Autodesk Inventor part; units mm, degrees
ref_plane "Work Plane1" through (0, 0, -9.525) normal (0, 0, -1) x (-1, 0, 0)
ref_plane "YZ Plane" through (0, 0, 0) normal (1, 0, 0) x (0, 1, 0)
ref_plane "XZ Plane" through (0, 0, 0) normal (0, 1, 0) x (-1, 0, 0)
sketch "Sketch1" plane through (0, 0, 0) normal (0, 0, 1) x (1, 0, 0)
  line L0 (-7.62, 3.048) -> (7.62, 3.048)
  line L1 (7.62, 3.048) -> (7.62, -3.048)
  line L2 (7.62, -3.048) -> (-7.62, -3.048)
  line L3 (-7.62, -3.048) -> (-7.62, 3.048)
  point P0 (0, 0)
  point P1 (0, -3.048)
  point P2 (-7.62, 0)
  dimension "d0" = 15.24
  dimension "d1" = 6.096
extrude "Extrusion1" add sketch "Sketch1" along normal blind 15.24
sketch "Sketch2" plane through (-7.62, 3.048, 0) normal (0, 1, 0) x (1, 0, 0)
  line L0 (0, -15.24) -> (15.24, -15.24)
  line L1 (2.54, -13.208) -> (12.7, -13.208)
  line L2 (12.7, -13.208) -> (12.7, -15.24)
  line L3 (12.7, -15.24) -> (2.54, -15.24)
  line L4 (2.54, -15.24) -> (2.54, -13.208)
  point P0 (7.62, -15.24)
  dimension "d4" = 10.16
  dimension "d5" = 2.032
extrude "Extrusion2" add sketch "Sketch2" along normal blind 1.27
sketch "Sketch3" plane through (-7.62, -3.048, 0) normal (0, -1, 0) x (1, 0, 0)
  line L0 (0, 15.24) -> (2.54, 15.24)
  line L1 (2.54, 15.24) -> (2.54, 13.208)
  line L2 (2.54, 13.208) -> (0, 13.208)
  line L3 (0, 13.208) -> (0, 15.24)
  line L4 (15.24, 15.24) -> (12.7, 15.24)
  line L5 (12.7, 15.24) -> (12.7, 13.208)
  line L6 (12.7, 13.208) -> (15.24, 13.208)
  line L7 (15.24, 13.208) -> (15.24, 15.24)
  dimension "d8" = 2.54
  dimension "d9" = 2.54
  dimension "d10" = 2.032
  dimension "d11" = 2.032
extrude "Extrusion3" add sketch "Sketch3" along normal blind 0.508
sketch "Sketch4" plane through (0, 0, 0) normal (0, 0, -1) x (-1, 0, 0)
  line L0 (7.62, 3.048) -> (-7.62, 3.048)
  line L1 (-7.62, 3.048) -> (-7.62, -3.048)
  line L2 (-7.62, -3.048) -> (7.62, -3.048)
  line L3 (7.62, -3.048) -> (7.62, 3.048)
  point P0 (-6.35, 1.27)
  point P1 (-3.81, 1.27)
  point P2 (3.81, 1.27)
  point P3 (6.35, 1.27)
  point P4 (-6.35, -1.27)
  point P5 (-3.81, -1.27)
  point P6 (3.81, -1.27)
  point P7 (6.35, -1.27)
  point P8 (0, 3.048)
  point P9 (-1.27, 1.27)
  point P10 (-1.27, -1.27)
  point P11 (1.27, 1.27)
  point P12 (1.27, -1.27)
  dimension "d14" = 1.27
  dimension "d15" = 1.778
  dimension "d16" = 1.27
  dimension "d17" = 1.778
  dimension "d18" = 2.54
  dimension "d19" = 2.54
  dimension "d20" = 2.54
  dimension "d21" = 2.54
ref_plane "Work Plane1" through (0, 0, -9.525) normal (0, 0, -1) x (-1, 0, 0)
sketch "Sketch5" plane through (0, 0, -9.525) normal (0, 0, -1) x (-1, 0, 0)
  point P0 (0, 0)
properties part number "12 Pin DR"
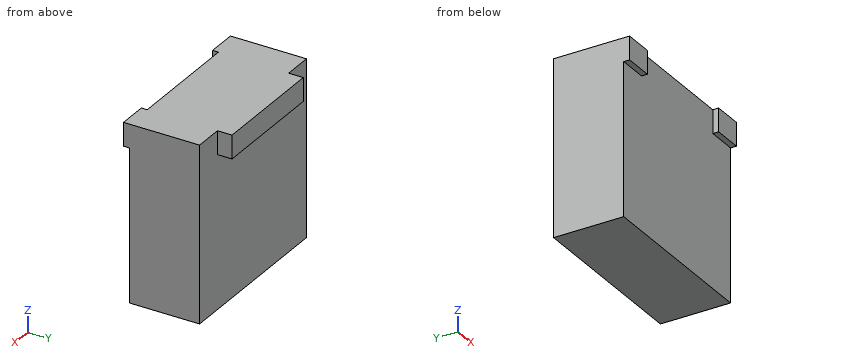
Work out the finished part from the listing and answer in its coordinate system (mm). Coordinates: 2 decimals unless noted, no trailing zeros. Loops run counter-clockwise (first coordinate to the right, second up) from the corner with the lowest first, then second, coordinate; pieces in that order, holes last. Notation, with made-up numbers: (-29.75, 53) - (-12.75, 53) arc R15 ccw to (-12.75, 72) - close; hole circle Ø6 at (-37, 75.5). An arc over 180 degrees is marked (long way). Use a Markdown table: item, result.
Item 1: Find section D-D, the plane z = 7. Determine the outline of the cut face in (x, y), and give its area (3 significant figures).
Evaluation:
| item | result |
|---|---|
| outline | (-7.62, -3.05) - (7.62, -3.05) - (7.62, 3.05) - (-7.62, 3.05) - close |
| area | 92.9 mm2 |
Item 2: Given pin 1 Ø3 at (x, y) = (-6, 2) entering from -Z; pin 2 Ø2 at (x, z) = (-1, 5.5) entering from -Y; pin 3 Ø0.6 at (y, z) = (3.5, 14) entering from -X; pin 4 Ø3 at (x, z) = (-5, 10) entering from +Y, each flat-ended and moving along its own axis, determine where each tip first touches the part or whether it passes through.
Evaluation:
| item | result |
|---|---|
| pin 1 | stops at z = 0 |
| pin 2 | stops at y = -3.05 |
| pin 3 | stops at x = -5.08 |
| pin 4 | stops at y = 3.05 |
Item 3: Find section C-C, the plane y = 3.75. Determine the outline of the cut face in (x, z).
Evaluation:
| item | result |
|---|---|
| outline | (-5.08, 13.21) - (5.08, 13.21) - (5.08, 15.24) - (-5.08, 15.24) - close |
Item 4: Find section B-B, the plane z = 14. Determine the outline of the cut face in (x, y).
Evaluation:
| item | result |
|---|---|
| outline | (-7.62, -3.56) - (-5.08, -3.56) - (-5.08, -3.05) - (5.08, -3.05) - (5.08, -3.56) - (7.62, -3.56) - (7.62, 3.05) - (5.08, 3.05) - (5.08, 4.32) - (-5.08, 4.32) - (-5.08, 3.05) - (-7.62, 3.05) - close |
Item 5: Consider probe 1 along Y at (x, z) = (6.75, 1.5); probe 2 along Z at (x, y) = (-2, 4.25). Determine where each line is inside the solid, lowest interval first. Write a range as from..to.
Evaluation:
| item | result |
|---|---|
| probe 1 | y = -3.05..3.05 |
| probe 2 | z = 13.21..15.24 |
Item 6: Find section A-A, the plane x = 6.25. Determine the outline of the cut face in (y, z), and give its area (3 significant figures).
Evaluation:
| item | result |
|---|---|
| outline | (-3.56, 13.21) - (-3.05, 13.21) - (-3.05, 0) - (3.05, 0) - (3.05, 15.24) - (-3.56, 15.24) - close |
| area | 93.9 mm2 |
